```python
from build123d import *

# Parameters (mm, degrees)
CROQUIS1_R              = 2
SALIENTE_EXTRUIR1_DEPTH = 5
CROQUIS2_W              = 5.3
CROQUIS2_H              = 38.303523839
CROQUIS2_W_2            = 18.5
CROQUIS2_H_2            = 11.2
CORTAR_EXTRUIR1_DEPTH   = 10


with BuildPart() as part:
    # Croquis1 → Saliente-Extruir1 (new body)
    with BuildSketch(Plane(origin=(0, 0, 0), x_dir=(0, 0, -1), z_dir=(1, 0, 0))):
        Polygon((0, 33.333333333), (5, 33.333333333), (5, 16.666666667), (0, 16.666666667), (0, 0), (30, 0), (30, 5), (60, 5), (60, 0), (90, 0), (90, 5), (120, 5), (120, 0), (150, 0), (150, 16.666666667), (145, 16.666666667), (145, 33.333333333), (150, 33.333333333), (150, 50), (120, 50), (120, 45), (90, 45), (90, 50), (60, 50), (60, 45), (30, 45), (30, 50), (0, 50), align=None)
        with Locations((16, 16)):
            Circle(CROQUIS1_R, mode=Mode.SUBTRACT)
        with Locations(Location((134, 16, 0), (0, 0, 180))):
            Circle(CROQUIS1_R, mode=Mode.SUBTRACT)
    extrude(amount=SALIENTE_EXTRUIR1_DEPTH)

    # Croquis2 → Cortar-Extruir1 (cut)
    with BuildSketch(Plane(origin=(5, 0, 0), x_dir=(0, 0, -1), z_dir=(1, 0, 0))):
        with Locations((10.65, 25.84823808)):
            Rectangle(CROQUIS2_W, CROQUIS2_H)
        with Locations((30.55, 35.4)):
            Rectangle(CROQUIS2_W_2, CROQUIS2_H_2)
    extrude(amount=-CORTAR_EXTRUIR1_DEPTH, mode=Mode.SUBTRACT)


solid = part.part
```
Geometry check sheet. Reference: the model listing, model coordinates, mm. A direction names the side the tool comes from. Coordinates: 2 decimals unless noted, no trailing zeros. Order: outer loops, then holes, each group sorted by start corner. A loop starts at its lowest first (then second) coordinate and runs counter-clockwise, first axis right, second up. Notation, with made-up numbers: (8, -1) - (60, -1) arc R27 cw to (60, 24) - close; hole circle Ø4 at (61.5, 64). An arc over 180 degrees is marked (long way). Answer as a JSON object with one key per item and string values. Group by question number.
Item 1: Sectioned sample at B-B, the plane y = 9. Record the cut outline in (x, z).
Item 2: Tool access check on faces 4 (the face through (2, 2, -90)), 5 (the face through (2, 45, -45)), 6 (the face through (3, 29.8, -30)). Record the directions out of +Z, -Z, +X, -X, +Y, -Y that give a thin tool (end or side, any length) a straight path to the whole face; none if there is none.
Item 3: Draft check along Y on faces 1 (the face through (2, 33.333, -2)), 2 (the face through (2, 50, -75)), 3 (the face through (2, 3, -120)). Enter one of: +Y half, -Y half, draft (parallel to the pull), parting line (faces both ways), or undercut.
Item 4: Scan lines: probe 1 along Z at (x, y) = (1.4, 4.5); probe 2 along Z at (x, y) = (3.1, 28.5); probe 3 along Z at (x, y) = (3.95, 30.5). Record each from-to range of solid material in increasing order.
Item 5: Sectioned sample at C-C, the plane x = 1.9. Give the number of separate pieces and of enclosed holes in the cut face, and give its area (3 significant figures).
Item 6: Sectioned sample at A-A, the plane z = -16. Record the cut outline in (x, y), and give its area (3 significant figures).
Item 7: Depth check by flat-ended pin: pin 1 Ø2 at (x, y) = (3, 21.5) entering from +Z; pin 2 Ø4.5 at (y, z) = (16, -16) entering from -X; pin 3 Ø1.5 at (x, z) = (1.5, -47.5) entering from +Y; pin 4 Ø2.5 at (x, y) = (3, 24) entering from -Z. Enter the tip coordinate at first touch or a pass-through.
Resolved:
{
 "1": {"outline": "(0, -150) - (5, -150) - (5, -13.3) - (0, -13.3) - close; (0, -8) - (5, -8) - (5, 0) - (0, 0) - close"},
 "2": {"face 4": "+X, -X, -Y", "face 5": "+X, -X, +Y", "face 6": "+X, -X"},
 "3": {"face 1": "undercut", "face 2": "+Y half", "face 3": "draft"},
 "4": {"probe 1": "-150 to -120, -90 to -60, -30 to 0", "probe 2": "-145 to -13.3, -8 to -5", "probe 3": "-145 to -39.8, -21.3 to -13.3, -8 to -5"},
 "5": {"separate pieces": "1", "enclosed holes": "4", "area": "6,300 mm^2"},
 "6": {"outline": "(0, 0) - (5, 0) - (5, 14) - (0, 14) - close; (0, 18) - (5, 18) - (5, 50) - (0, 50) - close", "area": "230 mm^2"},
 "7": {"pin 1": "z = -5", "pin 2": "x = 0", "pin 3": "y = 45", "pin 4": "z = -145"}
}
